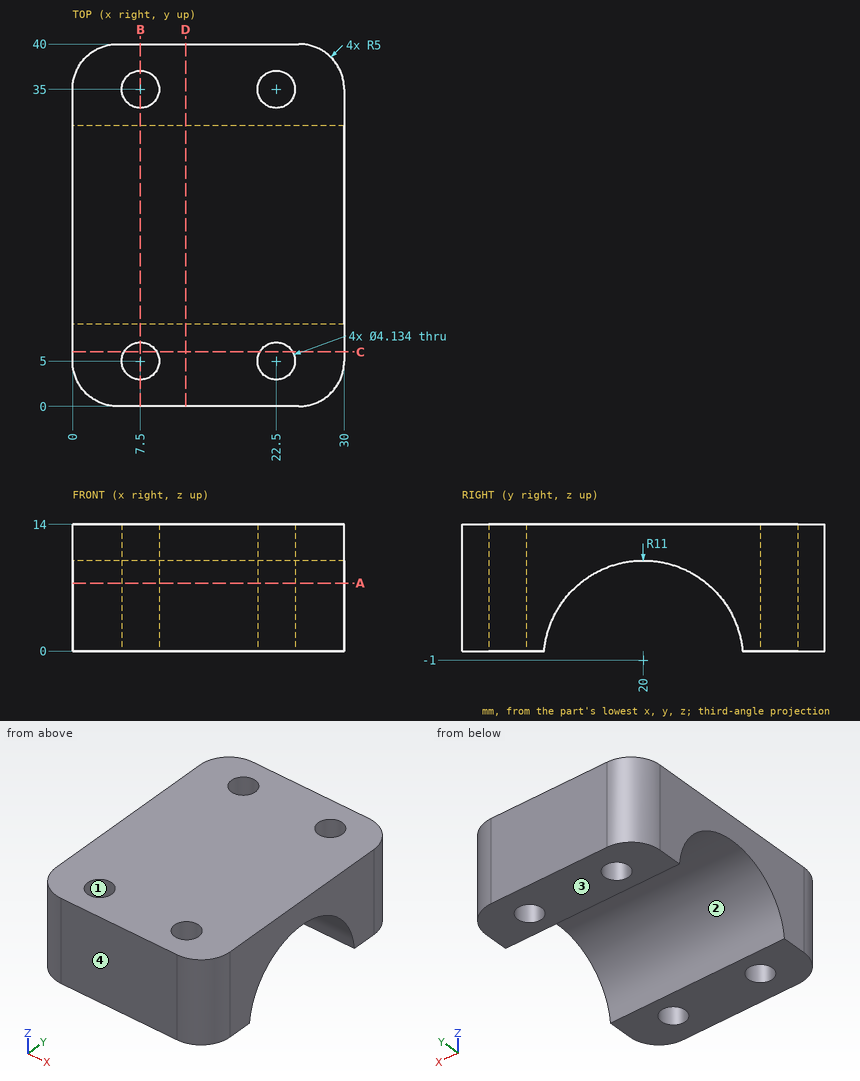
The drawing under review shows one solid part. Ordinate dimensions are in mm from its lowest x, y, z. Give positions to 0.01 mm unless a question says otherwise; leave off trailing zeros. Loops run counter-clockwise (first coordinate to the right, second up) from the corner with the lowest first, then second, coordinate; pieces in that order, holes last. Notation, with made-up numbers: M -15,70.25 L 39,70.25 A21 ccw 39,82.25 Z; hole C 5.25,-15 d3. An arc over 180 degrees is marked long. One line per question, with ' | ' between items. Start each with the question number.
1. Add section D-D (x = 12.5). Write out the cut boundary in (y, z), plus the area to 3 significant figures.
2. To check wall thickness, follow L1, parallel to X at y = 35, z = 11; L2, parallel to Y at x = 8.75, z = 6.25; L3, parallel to Y at x = 23.5, z = 2. State the ranges of each line that lie inside material, in increasing order.
3. Add section C-C (y = 6). Write out the cut boundary in (x, z).
4. Add section A-A (z = 7.5). Write out the cut boundary in (x, y), plus the area to 3 significant figures.
5. Add section B-B (x = 7.5). Write out the cut boundary in (y, z).
6. The part is to be moulded in two halves that separate along Y. For the marked faces 1, 2, 3 and 4, say which applies: released by +Y, released by -Y, zero draft, split by the parting line, or undercut.
Worked out:
1) outline: M 0,0 L 9.05,0 A11 cw 30.95,0 L 40,0 L 40,14 L 0,14 Z | area: 392 mm²
2) L1: x = 0 to 5.43, 9.57 to 20.43, 24.57 to 30 | L2: y = 0 to 3.35, 6.65 to 11.73, 28.27 to 33.35, 36.65 to 40 | L3: y = 0 to 3.19, 6.81 to 9.42, 30.58 to 33.19, 36.81 to 40
3) outline: M 0,0 L 5.69,0 L 5.69,14 L 0,14 Z; M 9.31,0 L 20.69,0 L 20.69,14 L 9.31,14 Z; M 24.31,0 L 30,0 L 30,14 L 24.31,14 Z
4) outline: M 0,5 A5 ccw 5,0 L 25,0 A5 ccw 30,5 L 30,13.02 L 0,13.02 Z; M 0,26.98 L 30,26.98 L 30,35 A5 ccw 25,40 L 5,40 A5 ccw 0,35 Z; hole C 7.5,5 d4.13; hole C 7.5,35 d4.13; hole C 22.5,5 d4.13; hole C 22.5,35 d4.13 | area: 706 mm²
5) outline: M 0,0 L 2.93,0 L 2.93,14 L 0,14 Z; M 7.07,0 L 9.05,0 A11 cw 30.95,0 L 32.93,0 L 32.93,14 L 7.07,14 Z; M 37.07,0 L 40,0 L 40,14 L 37.07,14 Z
6) face 1: undercut | face 2: undercut | face 3: zero draft | face 4: released by -Y
